Check sheet for the modelled part. Datum: model origin and axes. Units: mm. A direction names the side the tool comes from. Coordinates: 2 decimals unless noted, no trailing zeros. Write each loop counter-clockwise with the first axis right and the second up, starting at its lowest first coordinate (ties: lowest second). Pieces come first, ordered by that corner, then holes. Notation, with made-up numbers: M 21.5,-15.5 L 65.5,-15.5 A24 cw 65.5,-5.5 Z; hole C 87.5,-38 d10. An arc over 180 degrees is marked long. Answer as CSV lines item,"result".
from build123d import *

# Parameters (mm, degrees)
F0_W     = 8.6
F0_H     = 4.1
F0_W_2   = 9.2
F0_H_2   = 11.5
F1_DEPTH = 1.5
F2_D     = 5.2
F2_DEPTH = 2
F2_TIP   = 1.5622376095
F3_D     = 7
F3_DEPTH = 2
F3_TIP   = 2.1030121666
F4_D     = 5.3
F4_DEPTH = 2
F4_TIP   = 1.5922806404


with BuildPart() as f1:
    # F0 (on Top) → F1 (new body)
    with BuildSketch(Plane.XY):
        with BuildLine():
            Line((-37.75, -21), (37.75, -21))
            ThreePointArc((37.75, -21), (42.6997474683, -18.9497474683), (44.75, -14))
            Line((44.75, -14), (44.75, 14))
            ThreePointArc((44.75, 14), (42.6997474683, 18.9497474683), (37.75, 21))
            Line((37.75, 21), (-37.75, 21))
            ThreePointArc((-37.75, 21), (-42.6997474683, 18.9497474683), (-44.75, 14))
            Line((-44.75, 14), (-44.75, -14))
            ThreePointArc((-44.75, -14), (-42.6997474683, -18.9497474683), (-37.75, -21))
        make_face()
        with Locations((-5.25, -14.65)):
            Rectangle(F0_W, F0_H, mode=Mode.SUBTRACT)
        with Locations((-19.43, -5.25)):
            Rectangle(F0_W_2, F0_H_2, mode=Mode.SUBTRACT)
    extrude(amount=F1_DEPTH)

    # F2
    with Locations(Plane(origin=(0, 0, 0), x_dir=(1, 0, 0), z_dir=(0, 0, -1))):
        with Locations((18.75, 7), (-28.75, 7)):
            Hole(F2_D / 2, depth=F2_DEPTH)
            with Locations((0, 0, -(F2_DEPTH + F2_TIP / 2))):  # 118° drill point
                Cone(0, F2_D / 2, F2_TIP, mode=Mode.SUBTRACT)

    # F3
    with Locations(Plane(origin=(0, 0, 0), x_dir=(1, 0, 0), z_dir=(0, 0, -1))):
        with Locations((7.55, 7)):
            Hole(F3_D / 2, depth=F3_DEPTH)
            with Locations((0, 0, -(F3_DEPTH + F3_TIP / 2))):  # 118° drill point
                Cone(0, F3_D / 2, F3_TIP, mode=Mode.SUBTRACT)

    # F4
    with Locations(Plane(origin=(0, 0, 0), x_dir=(1, 0, 0), z_dir=(0, 0, -1))):
        with Locations((-30.2482247353, -5.4), (-30.2482247353, -15.4), (-21.9932247353, -15.4), (-21.9932247353, -5.4), (-13.7382247353, -15.4), (-13.7382247353, -5.4), (-5.4832247353, -15.4), (-5.4832247353, -5.4), (2.7717752647, -15.4), (2.7717752647, -5.4), (11.0267752647, -15.4), (11.0267752647, -5.4), (19.2817752647, -15.4), (19.2817752647, -5.4)):
            Hole(F4_D / 2, depth=F4_DEPTH)
            with Locations((0, 0, -(F4_DEPTH + F4_TIP / 2))):  # 118° drill point
                Cone(0, F4_D / 2, F4_TIP, mode=Mode.SUBTRACT)


solid = f1.part
1) Mould release check, pull along X, two halves, no side actions. Record for faces 1 (the face through (-42.65, 19, 0.74)), 2 (the face through (-1, 0, 1.5)), 3 (the face through (-19, -11, 1)): pulls with the +X half, pulls with the -X half, needs draft (parallel to the pull), parting line crosses it, or undercut.
Answer key:
face 1,"pulls with the -X half"
face 2,"needs draft"
face 3,"undercut"
2) Tool access check on faces 4 (the face through (-5, -12.6, 1)), 5 (the face through (1, 21, 1)). Record the directions out of +Z, -Z, +X, -X, +Y, -Y that give a thin tool (end or side, any length) a straight path to the whole face; none if there is none.
Answer key:
face 4,"+Z, -Z"
face 5,"+Z, -Z, +X, -X, +Y"
3) Depth check by flat-ended pin: P1, Ø0.8, axis at y = -15.5, z = 0.5, coming from the +X side; P2, Ø4, axis at x = 19.28, y = 5.4, coming from the -Z side. Enter the tip coordinate at first touch or a pass-through.
Answer key:
P1,"stops at x = 44.66"
P2,"passes through"
4) Section check C-C, the plane x = 7.55. Record the boundary of the cut face in (y, z).
Answer key:
outline,"M -21,0 L -10.5,0 L -10.5,1.5 L -21,1.5 Z; M -3.5,0 L 21,0 L 21,1.5 L -3.5,1.5 Z"
5) Section check D-D, the plane x = 18.75. Record the boundary of the cut face in (y, z), plus the area to 3 significant figures.
Answer key:
outline,"M -21,0 L -9.6,0 L -9.6,1.5 L -21,1.5 Z; M -4.4,0 L 2.8,0 L 2.8,1.5 L -4.4,1.5 Z; M 8,0 L 12.8,0 L 12.8,1.5 L 8,1.5 Z; M 18,0 L 21,0 L 21,1.5 L 18,1.5 Z"
area,"39.6 mm2"
6) Thickness scan on line 1 along Y through (x, z) = (-31.5, 1); line 2 along Y through (x, z) = (-30, 0.1); line 3 along X through (y, z) = (-10, 0.7). Record the ranges inside material, lowest first.
Answer key:
line 1,"y = -21 to 3.06, 7.74 to 13.06, 17.74 to 21"
line 2,"y = -21 to -9.28, -4.72 to 2.76, 8.04 to 12.76, 18.04 to 21"
line 3,"x = -44.75 to -24.03, -14.83 to 5.75, 9.35 to 44.75"
7) Section check A-A, the plane y = 5.4. Give the number of separate pieces and of enclosed holes in the cut face, plus the area to 3 significant figures.
Answer key:
separate pieces,"8"
enclosed holes,"0"
area,"78.6 mm2"
